CAD build for the part. Positions are in the model's coordinates, mm. Face numbers are marked on the shaded views. Give positions to 0.01 mm unless a question says otherwise; leave off trailing zeros. Order: outer loops, then holes, each group sorted by start corner. A loop starts at its lowest first (then second) coordinate and runs counter-clockwise, first axis right, second up.
Item 1: Band-saw the part on C-C on z = 114. Give the cut face in (x, y), plus the area to 3 significant figures.
Item 2: Two-plate mould, pull along Z, no slides. Class the marked faces 1, 2 and 3: released by +Z, released by -Z, zero draft, split by the parting line, or undercut.
Item 3: Band-saw the part on D-D on x = 27. Give the cut face in (y, z), plus the area to 3 significant figures.
Item 4: Band-saw the part on B-B on z = 53.5. Give the cut face in (x, y).
Item 5: Flat gauge pins, fed straight in: P1, Ø5, axis at x = -18, y = -20, coming from the +Z side; P2, Ø6, axis at x = 32.5, y = 20, coming from the +Z side. Where does each tip first touch, or does it go through?
Item 6: Wall check: L1, parallel to Z at x = 73, y = 0; L2, parallel to Z at x = -48, y = 0; L3, parallel to X at y = 16, z = 92.5. Give the ranges that are in metal, low to high.
Item 7: Band-saw the part on A-A on y = 0. Give the cut face in (x, z), plus the area to 3 significant figures.
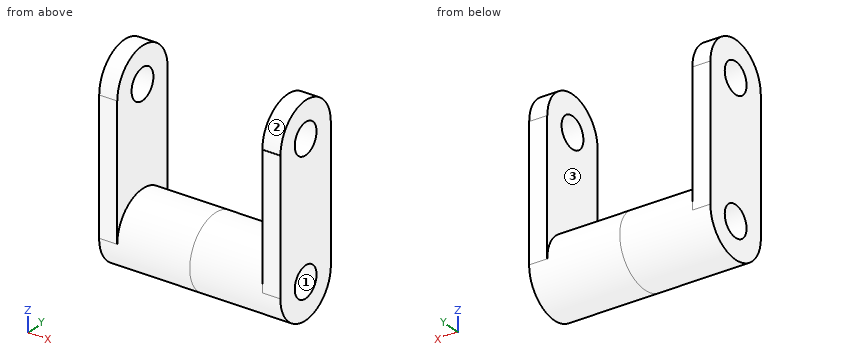
```python
from build123d import *

# Parameters (mm, degrees)
F0_R      = 31.646266
F1_DEPTH  = 80
F3_DEPTH  = 16
F4_R      = 31.533249
F5_DEPTH  = 16
F7_R      = 13.658774
F8_DEPTH  = 193
F9_R      = 13.658775
F10_DEPTH = 212


with BuildPart() as f1:
    # F0 (on Right) → F1 (new body)
    with BuildSketch(Plane.YZ):
        Circle(F0_R)
    extrude(amount=F1_DEPTH)

    # F2 (on face) → F3 (join)
    with BuildSketch(Plane.YZ.offset(80)):
        with BuildLine():
            Line((31.646266, 0), (31.646266, 117.492504))
            Line((31.646266, 117.492504), (-31.646266, 117.492504))
            Line((-31.646266, 117.492504), (-31.646266, 0))
            ThreePointArc((-31.646266, 0), (0, 31.646266), (31.646266, 0))
        make_face()
        with BuildLine():
            ThreePointArc((-31.646266, 0), (0, -31.646266), (31.646266, 0))
            Line((31.646266, 0), (-31.646266, 0))
        make_face()
    extrude(amount=-F3_DEPTH)

    # F4 (on face) → F5 (join)
    with BuildSketch(Plane.YZ.offset(80)):
        with Locations((0, 117.492504)):
            Circle(F4_R)
    extrude(amount=-F5_DEPTH)

    # F6: F1 across face


with BuildPart() as f1_1:
    add(f1.part)
    add(f1.part.mirror(Plane(origin=(0, 0, 0), x_dir=(0, 1, 0), z_dir=(-1, 0, 0))))

    # F7 (on face) → F8 (cut)
    with BuildSketch(Plane.YZ.offset(80)):
        Circle(F7_R)
    extrude(amount=-F8_DEPTH, mode=Mode.SUBTRACT)

    # F9 (on face) → F10 (cut)
    with BuildSketch(Plane.YZ.offset(80)):
        with Locations((0, 117.492504)):
            Circle(F9_R)
    extrude(amount=-F10_DEPTH, mode=Mode.SUBTRACT)


solid = f1_1.part
```
The answers:
1. outline: (-80, -31.65) - (-64, -31.65) - (-64, -13.2) - (-80, -13.2) - close; (-80, 13.2) - (-64, 13.2) - (-64, 31.65) - (-80, 31.65) - close; (64, -31.65) - (80, -31.65) - (80, -13.2) - (64, -13.2) - close; (64, 13.2) - (80, 13.2) - (80, 31.65) - (64, 31.65) - close
1. area: 1,180 mm2
2. face 1: undercut
2. face 2: released by +Z
2. face 3: zero draft
3. outline: circle Ø63.29 at (0, 0); hole circle Ø27.32 at (0, 0)
3. area: 2,560 mm2
4. outline: (-80, -31.65) - (-64, -31.65) - (-64, 31.65) - (-80, 31.65) - close; (64, -31.65) - (80, -31.65) - (80, 31.65) - (64, 31.65) - close
5. P1: stops at z = 26.37
5. P2: stops at z = 26.69
6. L1: z = -31.65 to -13.66, 13.66 to 103.83, 131.15 to 149.03
6. L2: z = -31.65 to -13.66, 13.66 to 31.65
6. L3: x = -80 to -64, 64 to 80
7. outline: (-80, -31.65) - (80, -31.65) - (80, -13.66) - (-80, -13.66) - close; (-80, 13.66) - (80, 13.66) - (80, 103.83) - (64, 103.83) - (64, 31.65) - (-64, 31.65) - (-64, 103.83) - (-80, 103.83) - close; (-80, 131.15) - (-64, 131.15) - (-64, 149.03) - (-80, 149.03) - close; (64, 131.15) - (80, 131.15) - (80, 149.03) - (64, 149.03) - close
7. area: 8,640 mm2
